CAD build for the part. Positions are in the model's coordinates, mm. A direction names the side the tool comes from. Round coordinates to 2 decimals unless told otherwise and drop trailing zeros. Loops run counter-clockwise (first coordinate to the right, second up) from the corner with the lowest first, then second, coordinate; pieces in that order, holes last. Notation, with made-up numbers: (66.25, 33) - (109.25, 33) arc R19 ccw to (109.25, 61) - close; hole circle Ø1 at (-34.75, 70.5). An arc over 180 degrees is marked (long way). Use one line per item in the form item = value.
from build123d import *

# Parameters (mm, degrees)
F0_W     = 12.7
F0_H     = 339.725
F1_DEPTH = 12.7


with BuildPart() as f1:
    # F0 (on Front) → F1 (new body)
    with BuildSketch(Plane.XZ):
        with BuildLine():
            Line((-241.3, 0), (-12.7, 0))
            Line((-12.7, 0), (-12.7, 339.725))
            Line((-12.7, 339.725), (-774.7, 339.725))
            Line((-774.7, 339.725), (-774.7, 0))
            Line((-774.7, 0), (-546.1, 0))
            Line((-546.1, 0), (-546.1, 234.95))
            ThreePointArc((-546.1, 234.95), (-527.501281, 279.851281), (-482.6, 298.45))
            Line((-482.6, 298.45), (-393.7, 298.45))
            Line((-393.7, 298.45), (-304.8, 298.45))
            ThreePointArc((-304.8, 298.45), (-259.898719, 279.851281), (-241.3, 234.95))
            Line((-241.3, 234.95), (-241.3, 0))
        make_face()
        with Locations((-6.35, 169.8625)):
            Rectangle(F0_W, F0_H)
        with Locations((-781.05, 169.8625)):
            Rectangle(F0_W, F0_H)
    extrude(amount=F1_DEPTH)


solid = f1.part
1) Flat gauge pin, fed straight in: pin 1 (6.5 mm diameter, centred on x = -364, y = -5, fed in from -Z). Where does the tip first touch, or does it go through?
Report:
pin_1 = 298.45
2) Slice it at C-C (x = -335). Write the cut outline in (y, z) (3 decimals).
Report:
outline = (-12.7, 298.45) - (0, 298.45) - (0, 339.725) - (-12.7, 339.725) - close
3) Slice it at A-A (z = 70). Write the cut outline in (x, y).
Report:
outline = (-787.4, -12.7) - (-546.1, -12.7) - (-546.1, 0) - (-787.4, 0) - close; (-241.3, -12.7) - (0, -12.7) - (0, 0) - (-241.3, 0) - close
4) Slice it at B-B (y = -2.25). Write the cut outline in (x, z) (3 decimals).
Report:
outline = (-787.4, 0) - (-546.1, 0) - (-546.1, 234.95) arc R63.5 cw to (-482.6, 298.45) - (-304.8, 298.45) arc R63.5 cw to (-241.3, 234.95) - (-241.3, 0) - (0, 0) - (0, 339.725) - (-787.4, 339.725) - close
5) Tool access for faces 3 (the flat face through (-399, -12.7, 323)), 4 (the cylindrical face through (-527.992, -6.261, 279.355)): list every direction of +Z, -Z, +X, -X, +Y, -Y with a clear straight run to the whole face (end or side of a thin tool).
Report:
face_3 = +Z, -Z, +X, -X, -Y
face_4 = -Z, +Y, -Y
6) Slice it at D-D (z = 272.5). Write the cut outline in (x, y), plus the area to 3 significant figures.
Report:
outline = (-787.4, -12.7) - (-533.81, -12.7) - (-533.81, 0) - (-787.4, 0) - close; (-253.59, -12.7) - (0, -12.7) - (0, 0) - (-253.59, 0) - close
area = 6,440 mm^2
7) Drill centre lines: probe 1 along X at (y, z) = (-10, 196.5); probe 2 along Z at (x, y) = (-321, -8) (3 decimals); probe 3 along X at (y, z) = (-8.25, 282). Where is each one in solid material? Low to high.
Report:
probe_1 = -787.4 to -546.1, -241.3 to 0
probe_2 = 298.45 to 339.725
probe_3 = -787.4 to -525.24, -262.16 to 0
8) Two-plate mould, pull along X, no slides. Class faces 1 (the flat face through (-399, 0, 323)), 2 (the cylindrical face through (-260.395, -6.261, 280.342)): +X half, -X half, draft (parallel to the pull), parting line (faces both ways), or undercut.
Report:
face_1 = draft
face_2 = undercut
